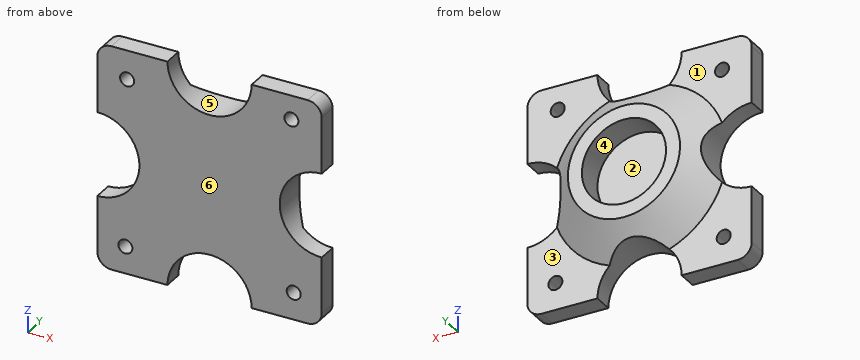
```python
from build123d import *

# Parameters (mm, degrees)
BOSS_EXTRUDE1_DEPTH = 8.89
SKETCH3_R           = 19.05
SKETCH3_R_2         = 3.175
CUT_EXTRUDE5_DEPTH  = 59.944
SKETCH3_9_R         = 19.05
SKETCH3_9_R_2       = 3.175
CUT_EXTRUDE7_DEPTH  = 71.374
SKETCH3_12_R        = 19.05
BOSS_EXTRUDE2_DEPTH = 8.89


with BuildPart() as part:
    # Sketch1 → Boss-Extrude1 (new body)
    with BuildSketch(Plane(origin=(0, 0, 0), x_dir=(1, 0, 0), z_dir=(0, 1, 0))):
        with BuildLine():
            Line((-44.45, 50.8), (44.45, 50.8))
            ThreePointArc((44.45, 50.8), (48.940128061, 48.940128061), (50.8, 44.45))
            Line((50.8, 44.45), (50.8, -44.45))
            ThreePointArc((50.8, -44.45), (48.940128061, -48.940128061), (44.45, -50.8))
            Line((44.45, -50.8), (-44.45, -50.8))
            ThreePointArc((-44.45, -50.8), (-48.940128061, -48.940128061), (-50.8, -44.45))
            Line((-50.8, -44.45), (-50.8, 44.45))
            ThreePointArc((-50.8, 44.45), (-48.940128061, 48.940128061), (-44.45, 50.8))
        make_face()
    extrude(amount=BOSS_EXTRUDE1_DEPTH)

    # Sketch2 → Revolve1 (revolve)
    with BuildSketch(Plane.XY, mode=Mode.PRIVATE) as revolve1_sk:
        Polygon((0, 0), (0, 21.59), (25.4, 21.59), (41.275, 7.544465781), align=None)
    revolve(revolve1_sk.sketch.rotate(Axis((0, 0, 0), (0, 1, 0)), 90), axis=Axis((0, 0, 0), (0, 1, 0)))

    # Sketch3 → Cut-Extrude5 (cut)
    with BuildSketch(Plane(origin=(0, 0, 0), x_dir=(1, 0, 0), z_dir=(0, 1, 0))):
        with Locations((-50.8, 0)):
            Circle(SKETCH3_R)
        with Locations((50.8, 0)):
            Circle(SKETCH3_R)
        with Locations((0, 50.8)):
            Circle(SKETCH3_R)
        with Locations((0, -50.8)):
            Circle(SKETCH3_R)
        with Locations(Location((-38.1, 38.550826986, 0), (0, 0, 270))):
            Circle(SKETCH3_R_2)
        with Locations(Location((38.1, 38.550826986, 0), (0, 0, 270))):
            Circle(SKETCH3_R_2)
        with Locations(Location((37.0502476, -39.95194326, 0), (0, 0, 270))):
            Circle(SKETCH3_R_2)
        with Locations(Location((-37.332084064, -37.649173014, 0), (0, 0, 270))):
            Circle(SKETCH3_R_2)
    extrude(amount=CUT_EXTRUDE5_DEPTH, mode=Mode.SUBTRACT)

    # Sketch3<9> → Cut-Extrude7 (cut)
    with BuildSketch(Plane(origin=(0, 0, 0), x_dir=(1, 0, 0), z_dir=(0, 1, 0))):
        with Locations((-50.8, 0)):
            Circle(SKETCH3_9_R)
        with Locations(Location((0, 0, 0), (0, 0, 270))):
            Circle(SKETCH3_9_R)
        with Locations((50.8, 0)):
            Circle(SKETCH3_9_R)
        with Locations((0, 50.8)):
            Circle(SKETCH3_9_R)
        with Locations((0, -50.8)):
            Circle(SKETCH3_9_R)
        with Locations(Location((-38.1, 38.550826986, 0), (0, 0, 270))):
            Circle(SKETCH3_9_R_2)
        with Locations(Location((38.1, 38.550826986, 0), (0, 0, 270))):
            Circle(SKETCH3_9_R_2)
        with Locations(Location((37.0502476, -39.95194326, 0), (0, 0, 270))):
            Circle(SKETCH3_9_R_2)
        with Locations(Location((-37.332084064, -37.649173014, 0), (0, 0, 270))):
            Circle(SKETCH3_9_R_2)
    extrude(amount=CUT_EXTRUDE7_DEPTH, mode=Mode.SUBTRACT)

    # Sketch3<12> → Boss-Extrude2 (add)
    with BuildSketch(Plane(origin=(0, 0, 0), x_dir=(1, 0, 0), z_dir=(0, 1, 0))):
        with Locations(Location((0, 0, 0), (0, 0, 270))):
            Circle(SKETCH3_12_R)
    extrude(amount=BOSS_EXTRUDE2_DEPTH)


solid = part.part
```
CAD build for the part. Positions are in the model's coordinates, mm. Face numbers are marked on the shaded views. A direction names the side the tool comes from. Round coordinates to 2 decimals unless told otherwise and drop trailing zeros. Order: outer loops, then holes, each group sorted by start corner. A loop starts at its lowest first (then second) coordinate and runs counter-clockwise, first axis right, second up. Notation, with made-up numbers: (27.25, 4) - (80.25, 4) arc R25 cw to (80.25, 26) - close; hole circle Ø5 at (-29.75, 6). An arc over 180 degrees is marked (long way). Answer in a Markdown table with one row per item. Add a question column.
(1) Mould opens along Z. For the marked faces 4, 5 and 6 say: +Z half, -Z half, draft (parallel to the pull), parting line (faces both ways), or undercut.
(2) Band-saw the part on B-B on y = 5.5. List the corners of the cut face in (x, z) (3 decimals), and give its area (3 significant figures).
(3) 3-axis set-ups, long thin cutter, end or side, ignore diameter. For the marked faces 1, 2 and 3: which of +Z, -Z, +X, -X, +Y, -Y reach the whole face in a straight line?
(4) Probe L1, parallel to Z at x = 0, y = 13.5; L2, parallel to Z at x = 38.1, y = 2.25; L3, parallel to Y at x = 34, z = 22.5. List the from-to ranges inside material, lowest first. Write a range as [from, to].
(5) Band-saw the part on A-A on x = 0. List the corners of the cut face in (y, z).
(6) Drop flat-ended pins along their axis: pin 1 Ø10 at (x, y) = (3.5, 3.5) entering from +Z; pin 2 Ø5 at (x, z) = (37.05, 39.95) entering from +Y; pin 3 Ø10 at (x, y) = (-0.5, 16) entering from -Z; pin 4 Ø8 at (y, z) = (19, -19) entering from -X. Give the stop position or say it passes through.
Data:
| question | item | result |
|---|---|---|
| 1 | face 4 | undercut |
| 1 | face 5 | +Z half |
| 1 | face 6 | draft |
| 2 | outline | (-50.8, -44.45) arc R6.35 ccw to (-44.45, -50.8) - (-19.05, -50.8) arc R19.05 cw to (19.05, -50.8) - (44.45, -50.8) arc R6.35 ccw to (50.8, -44.45) - (50.8, -19.05) arc R19.05 cw to (50.8, 19.05) - (50.8, 44.45) arc R6.35 ccw to (44.45, 50.8) - (19.05, 50.8) arc R19.05 cw to (-19.05, 50.8) - (-44.45, 50.8) arc R6.35 ccw to (-50.8, 44.45) - (-50.8, 19.05) arc R19.05 cw to (-50.8, -19.05) - close; hole circle Ø6.35 at (-38.1, -38.551); hole circle Ø6.35 at (-37.332, 37.649); hole circle Ø6.35 at (37.05, 39.952); hole circle Ø6.35 at (38.1, -38.551) |
| 2 | area | 7,880 mm^2 |
| 3 | face 1 | +Z, -X, +Y |
| 3 | face 2 | +Y |
| 3 | face 3 | -Z, +X, +Y |
| 4 | L1 | z = [-31.75, -19.05], [19.05, 31.75] |
| 4 | L2 | z = [-50.8, -41.73], [-35.38, -14.2], [14.2, 36.96], [42.95, 50.8] |
| 4 | L3 | y = [0, 8.89] |
| 5 | outline | (0, -31.75) - (15.97, -31.75) - (21.59, -25.4) - (21.59, -19.05) - (8.89, -19.05) - (8.89, 19.05) - (21.59, 19.05) - (21.59, 25.4) - (15.97, 31.75) - (0, 31.75) - close |
| 6 | pin 1 | stops at z = 33.75 |
| 6 | pin 2 | passes through |
| 6 | pin 3 | stops at z = -32.52 |
| 6 | pin 4 | stops at x = -27.42 |
